Verification items for the finished model (mm, model axes). Face numbers are marked on the shaded views. A direction names the side the tool comes from. Give positions to 0.01 mm unless a question says otherwise; leave off trailing zeros. Write each loop counter-clockwise with the first axis right and the second up, starting at its lowest first coordinate (ties: lowest second). Pieces come first, ordered by that corner, then holes.
Autodesk Inventor part; units mm, degrees
ref_plane "YZ Plane" through (0, 0, 0) normal (1, 0, 0) x (0, 1, 0)
ref_plane "XZ Plane" through (0, 0, 0) normal (0, 1, 0) x (-1, 0, 0)
ref_plane "XY Plane" through (0, 0, 0) normal (0, 0, 1) x (1, 0, 0)
sketch "Skizze1" plane through (0, 0, 0) normal (1, 0, 0) x (0, 1, 0)
  arc A0 (-7.2187, 8.3) -> (7.2187, 8.3) centre (0, 0) ccw construction
  line L0 (14, 8.3) -> (-14, 8.3)
  line L1 (-14, 8.3) -> (-14, 1.8)
  line L2 (0, 12.16) -> (0, -14.86)
  circle A1 centre (0, 0) radius 5
  line L3 (14, 0.3) -> (14, 8.3)
  line L4 (-14, 1.8) -> (-2, -11)
  line L5 (-2, -11) -> (5.4841, -11)
  line L6 (5.4841, -11) -> (14, 0.3)
  circle A2 centre (10.504, 0.982) radius 1.525
  dimension "d0" = 22
  dimension "d2" = 10
  dimension "d19" = 8.3
  dimension "d39" = 14
  dimension "d50" = 3.05
  dimension "d57" = 10.504
  dimension "d61" = 2
  dimension "d62" = 6.5
  dimension "d63" = 8
  dimension "d86" = 10.5498
  dimension "d87" = 7.318
  dimension "d88" = 0.982
extrude "Extrusion1" add sketch "Skizze1" along normal mid plane 6 contours L3 L6 L5 L2 A1 L0 | L2 A1 L5 L4 L1 L0
sketch "Skizze2" plane through (3, 0, 0) normal (1, 0, 0) x (0, 0, -1)
  circle A0 centre (0, 0) radius 8.5 construction
  line L0 (0, 0) -> (8.5, 0) construction
  line L1 (-12.4, 0) -> (14.9, 0)
  dimension "d6" = 17
hole "Bohrung1" at (3, 0, -8.5) direction (-1, 0, 0) diameter 2.1 end through all counterbore diameter 4.2 counterbore depth 2.8
pattern_circular "Runde Anordnung1" count 3 over 360 about axis through (0, 0, 0) along (1, 0, 0) of "Bohrung1"
sketch "Skizze3" plane through (-3, -14, 8.3) normal (0, 0, 1) x (1, 0, 0)
  line L0 (0, 0) -> (6, 0)
  line L1 (6, 28) -> (6, 0)
  line L2 (0, 0) -> (0, 28)
  line L3 (0, 0) -> (6, 0) construction
  line L4 (3, 0) -> (3, 24.0467) construction
  line L5 (6, 28) -> (0, 28)
  line L6 (-1.2, 14) -> (7.2, 14)
  point P0 (3, 14)
  point P1 (3, 3)
  point P2 (3, 25)
  dimension "d44" = 11
hole "Bohrung2" at (0, -11, 8.3) at (0, 11, 8.3) direction (0, 0, -1) diameter 2.459 depth 6 tip angle 118
fillet "Rundung2" radius 2 4 edges at (0, -2, -11) (0, 5.4841, -11) (0, -14, 1.8) (0, 14, 0.3)
sketch "Skizze7" plane through (-3, -14, 8.3) normal (0, 0, 1) x (1, 0, 0)
  line L0 (3, 33.6) -> (3, -5.6) construction
  line L1 (-1.2, 14) -> (7.2, 14) construction
  point P0 (3, 14)
  point P1 (3, 10)
  point P2 (3, 18)
  dimension "d78" = 8
hole "Bohrung4" [suppressed]
sketch "Skizze6" plane through (3, 0, 0) normal (1, 0, 0) x (0, 0, -1)
  circle A0 centre (0.5, -7.5) radius 1.5
  circle A1 centre (0.5, -7.5) radius 3 construction
  circle A2 centre (-0.982, 10.504) radius 1.525 construction
  circle A3 centre (-0.982, 10.504) radius 2.75 construction
  circle A4 centre (3, 7.5) radius 3 construction
  circle A5 centre (3, 7.5) radius 1.5
  line L0 (-1.223, -13.4591) -> (10.3679, -2.5926) construction
  line L1 (10.2037, 6.0842) -> (0.2345, 13.5972) construction
  circle A6 centre (-4.25, -7.3612) radius 2.1 construction
  circle A7 centre (0, 0) radius 5 construction
  dimension "d64" = 3
  dimension "d65" = 6
  dimension "d66" = 5.5
  dimension "d67" = 6
  dimension "d68" = 3
  dimension "d69" = 1.152
  dimension "d70" = 1.963
  dimension "d71" = 7.5
  dimension "d72" = 0.5
  dimension "d73" = 7.5
  dimension "d74" = 3
  dimension "d75" = 1.0167
extrude "Fräshalterung Schrauben" [suppressed]
properties part number "Motorhalter" material "Aluminium 6061"
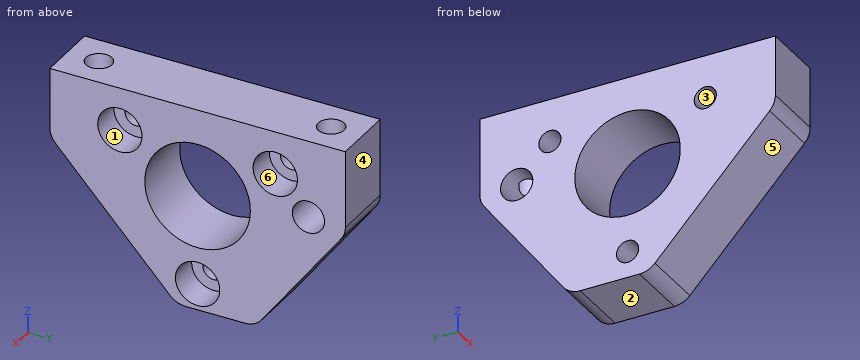
Item 1: Depth check by flat-ended pin: pin 1 (2 mm diameter, centred on x = -1.5, z = 0, fed in from -Y); pin 2 (2.5 mm diameter, centred on y = 7.36, z = 4.25, fed in from +X); pin 3 (1.3 mm diameter, centred on y = 0, z = -8.5, fed in from +X). Enter the tip coordinate at first touch or a pass-through.
Answer key:
pin 1: stops at y = -13.25
pin 2: stops at x = 0.2
pin 3: passes through
Item 2: Sectioned sample at A-A on z = 4.25. Record the cut outline in (x, y).
Answer key:
outline: (-3, -14) - (3, -14) - (3, -9.46) - (0.2, -9.46) - (0.2, -8.41) - (-3, -8.41) - close; (-3, -6.31) - (0.2, -6.31) - (0.2, -5.26) - (3, -5.26) - (3, -2.63) - (-3, -2.63) - close; (-3, 2.63) - (3, 2.63) - (3, 5.26) - (0.2, 5.26) - (0.2, 6.31) - (-3, 6.31) - close; (-3, 8.41) - (0.2, 8.41) - (0.2, 9.46) - (3, 9.46) - (3, 14) - (-3, 14) - close; hole circle Ø2.46 at (0, -11); hole circle Ø2.46 at (0, 11)
Item 3: Release check for a two-part mould opening along Y. For the marked faces 1, 2, 3 and 4 record: released by +Y, released by -Y, zero draft, split by the parting line, or undercut.
Answer key:
face 1: undercut
face 2: zero draft
face 3: undercut
face 4: released by +Y
Item 4: Sectioned sample at C-C on x = 2. Record the cut outline in (y, z) (3 decimals).
Answer key:
outline: (-14, 2.591) arc R2 ccw to (-13.459, 1.223) - (-2.593, -10.368) arc R2 ccw to (-1.134, -11) - (4.487, -11) arc R2 ccw to (6.084, -10.204) - (13.597, -0.234) arc R2 ccw to (14, 0.969) - (14, 8.3) - (-14, 8.3) - close; hole circle Ø4.2 at (-7.361, 4.25); hole circle Ø10 at (0, 0); hole circle Ø4.2 at (0, -8.5); hole circle Ø4.2 at (7.361, 4.25); hole circle Ø3.05 at (10.504, 0.982)
Item 5: Sectioned sample at D-D on z = -4. Record the cut outline in (x, y), then the cut area to 3 significant figures.
Answer key:
outline: (-3, -8.56) - (3, -8.56) - (3, -3) - (-3, -3) - close; (-3, 3) - (3, 3) - (3, 10.76) - (-3, 10.76) - close
area: 79.9 mm2
Item 6: Sectioned sample at B-B on z = -8.5. Record the cut outline in (x, y).
Answer key:
outline: (-3, -4.34) - (3, -4.34) - (3, -2.1) - (0.2, -2.1) - (0.2, -1.05) - (-3, -1.05) - close; (-3, 1.05) - (0.2, 1.05) - (0.2, 2.1) - (3, 2.1) - (3, 7.37) - (-3, 7.37) - close
Item 7: Set-up check for the marked faces 5 and 6: record each of +Z, -Z, +X, -X, +Y, -Y from which the full face is reachable in a straight line by a thin tool's end or side.
Answer key:
face 5: -Z, +X, -X, -Y
face 6: +X
Item 8: Scan lines: line 1 along Z through (x, y) = (-2.1, 0); line 2 along Y through (x, z) = (0.5, 2); line 3 along Y through (x, z) = (2.5, 0). Record each from-to range of solid material in increasing order.
Answer key:
line 1: z = -11 to -9.55, -7.45 to -5, 5 to 8.3
line 2: y = -13.91 to -11.53, -10.47 to -4.58, 4.58 to 9.37, 11.64 to 14
line 3: y = -12.31 to -5, 5 to 9.34, 11.67 to 13.75
